Could you check a few things on this drawing? It's one solid part, dimensions in mm from its lowest x, y, z. A direction names the side the tool comes from. Round coordinates to 2 decimals unless told otherwise and drop trailing zeros. Write each loop counter-clockwise with the first axis right and the second up, starting at its lowest first coordinate (ties: lowest second). Pieces come first, ordered by that corner, then holes. Notation, with made-up numbers: (32, -0.75) -> (41, -0.75) arc R20 cw to (41, 15.25) -> close; hole circle Ø1 at (84, 60.25). An arc over 180 degrees is marked (long way). Return JSON: item names as keys, results as strings.
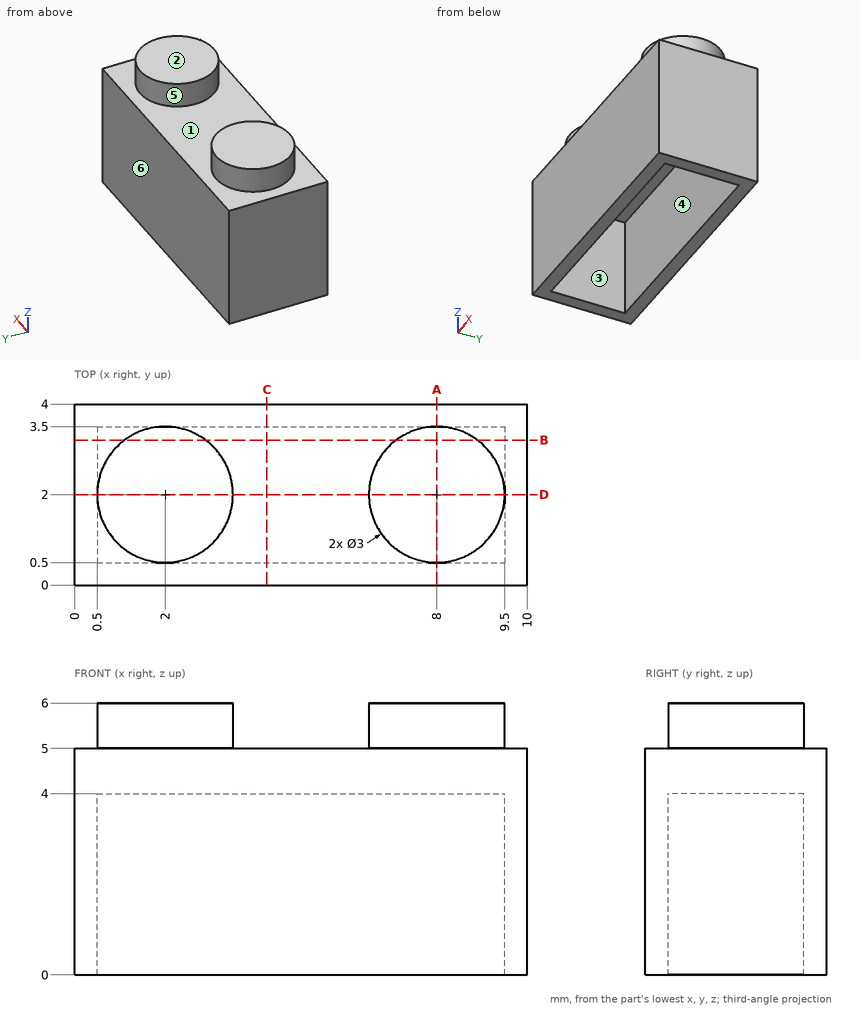
1) I want a section at C-C, the plane x = 4.25. Please give me the cut outline in (y, z).
Return value:
{"outline": "(0, 0) -> (0.5, 0) -> (0.5, 4) -> (3.5, 4) -> (3.5, 0) -> (4, 0) -> (4, 5) -> (0, 5) -> close"}
2) For the marked faces 1, 2 and 3, which set-ups out of +Z, -Z, +X, -X, +Y, -Y let a thin tool reach every point of the face, with its end or its side?
Return value:
{"face 1": "+Z", "face 2": "+Z, +X, -X, +Y, -Y", "face 3": "-Z"}
3) If I drill on probe 1 along Y at (x, z) = (7, 1.7); probe 2 along X at (y, z) = (0.85, 1.25); probe 3 along Z at (x, y) = (4, 0.8), over which ranges is the centre line in solid material (lowest first)? Write a range as [from, to].
Return value:
{"probe 1": "[0, 0.5], [3.5, 4]", "probe 2": "[0, 0.5], [9.5, 10]", "probe 3": "[4, 5]"}
4) Thinking about a two-plate mould opening in Y: for the marked faces 4, 5 and 6, which applies, pulls with the +Y half, pulls with the -Y half, needs draft (parallel to the pull), parting line crosses it, or undercut?
Return value:
{"face 4": "undercut", "face 5": "parting line crosses it", "face 6": "pulls with the +Y half"}
5) Will these pins go through, and if not, where does the flat tip stop? pin 1 Ø3 at (x, z) = (4, 1) entering from -Y; pin 2 Ø0.9 at (x, y) = (3.5, 1.5) entering from -Z.
Return value:
{"pin 1": "y = 0", "pin 2": "z = 4"}
6) I want a section at B-B, the plane y = 3.2. Please give me the cut outline in (x, z), and give its area (3 significant figures).
Return value:
{"outline": "(0, 0) -> (0.5, 0) -> (0.5, 4) -> (9.5, 4) -> (9.5, 0) -> (10, 0) -> (10, 5) -> (8.9, 5) -> (8.9, 6) -> (7.1, 6) -> (7.1, 5) -> (2.9, 5) -> (2.9, 6) -> (1.1, 6) -> (1.1, 5) -> (0, 5) -> close", "area": "17.6 mm²"}
7) I want a section at A-A, the plane x = 8. Please give me the cut outline in (y, z), and give its area (3 significant figures).
Return value:
{"outline": "(0, 0) -> (0.5, 0) -> (0.5, 4) -> (3.5, 4) -> (3.5, 0) -> (4, 0) -> (4, 5) -> (3.5, 5) -> (3.5, 6) -> (0.5, 6) -> (0.5, 5) -> (0, 5) -> close", "area": "11.0 mm²"}
8) I want a section at D-D, the plane y = 2. Please give me the cut outline in (x, z), and give its area (3 significant figures).
Return value:
{"outline": "(0, 0) -> (0.5, 0) -> (0.5, 4) -> (9.5, 4) -> (9.5, 0) -> (10, 0) -> (10, 5) -> (9.5, 5) -> (9.5, 6) -> (6.5, 6) -> (6.5, 5) -> (3.5, 5) -> (3.5, 6) -> (0.5, 6) -> (0.5, 5) -> (0, 5) -> close", "area": "20.0 mm²"}
